Input: dimensioned drawing with shaded views. Units: mm. Origin: part minimum x, y, z. A direction names the side the tool comes from. Coordinates: 2 decimals unless noted, no trailing zeros. Loops run counter-clockwise (first coordinate to the right, second up) from the corner with the lowest first, then second, coordinate; pieces in that order, holes last. Notation, with made-up numbers: (-13, -15) - (14, -15) arc R28 ccw to (14, 24) - close; hole circle Ø2 at (-7.75, -6.5). An arc over 180 degrees is marked (long way). Put each result on its own line as item: value. Start each with the question number.
1) Material intervals for line 1 along Z through (x, y) = (80.5, 5); line 2 along Y through (x, z) = (30, 33); line 3 along Z through (x, y) = (34.5, 27.5), sorted ascending. Write a range as from..to.
2) Reachability of the marked faces 4 and 5 from +Z, -Z, +X, -X, +Y, -Y: full face, straight path, thin tool, end or side. Return the list, or none.
3) Section A-A on y = 8.5. Output: boundary loops of the cut face in (x, z), and give its area (3 significant figures).
4) Section C-C on z = 15. Output: boundary loops of the cut face in (x, y), and give its area (3 significant figures).
5) Section D-D on x = 47. Output: boundary loops of the cut face in (y, z).
6) Contact query for flat-ended pins moving along their axis: pin 1 Ø12 at (x, y) = (17, 27.5) entering from -Z; pin 2 Ø13 at (x, z) = (26, 29) entering from -Y; pin 3 Ø1.5 at (y, z) = (10, 43.5) entering from -X; pin 4 Ø8 at (x, z) = (41.5, 9.5) entering from +Y. Output: stop coordinate, or through.
7) Draft query along Z for the marked faces 1, 2 and 3. Return one class per face: +Z half, -Z half, draft (parallel to the pull), parting line (faces both ways), or undercut.
8) Section B-B on x = 15.5. Output: boundary loops of the cut face in (y, z), and give its area (3 significant figures).
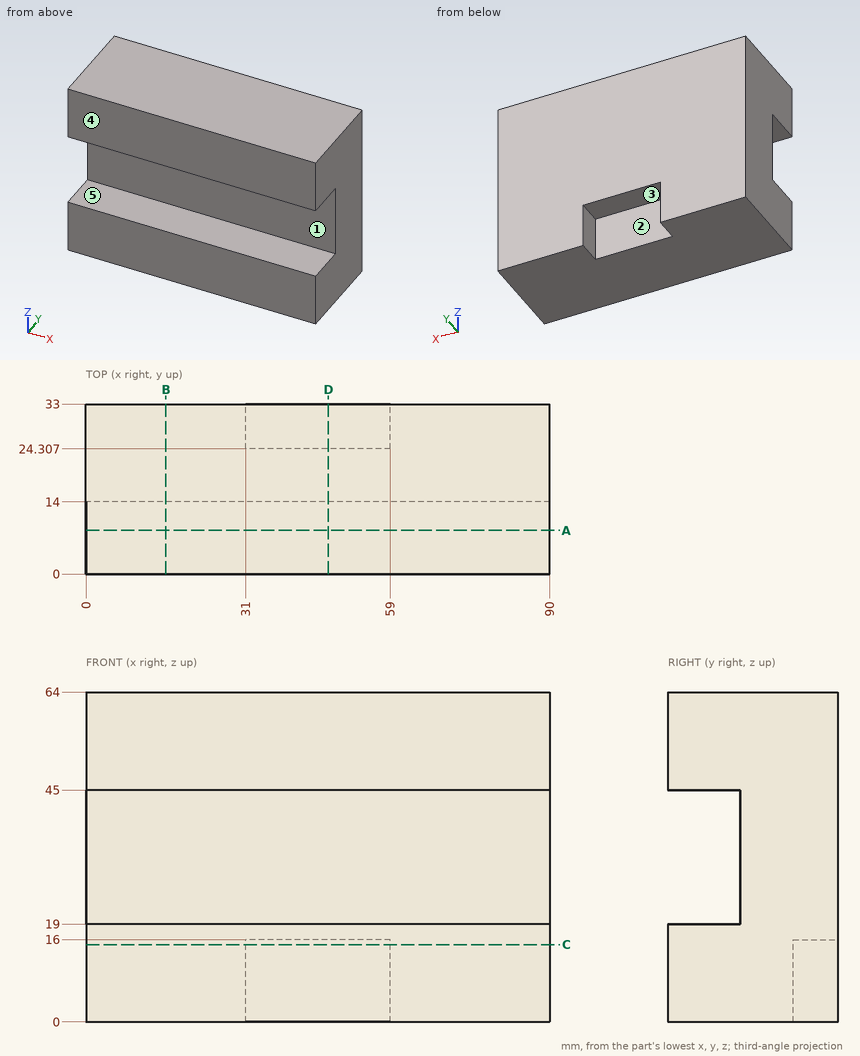
Answer block:
1. line 1: z = 0..19, 45..64
1. line 2: y = 14..33
1. line 3: z = 16..64
2. face 4: +Z, -Z, +X, -X, -Y
2. face 5: +X, -X, -Y
3. outline: (0, 0) - (90, 0) - (90, 19) - (0, 19) - close; (0, 45) - (90, 45) - (90, 64) - (0, 64) - close
3. area: 3,420 mm²
4. outline: (0, 0) - (90, 0) - (90, 33) - (59, 33) - (59, 24.31) - (31, 24.31) - (31, 33) - (0, 33) - close
4. area: 2,730 mm²
5. outline: (0, 0) - (24.31, 0) - (24.31, 16) - (33, 16) - (33, 64) - (0, 64) - (0, 45) - (14, 45) - (14, 19) - (0, 19) - close
6. pin 1: stops at z = 0
6. pin 2: stops at y = 14
6. pin 3: passes through
6. pin 4: stops at y = 24.31
7. face 1: undercut
7. face 2: draft
7. face 3: -Z half
8. outline: (0, 0) - (33, 0) - (33, 64) - (0, 64) - (0, 45) - (14, 45) - (14, 19) - (0, 19) - close
8. area: 1,750 mm²
